Part model, mm, in its own coordinate system. Face numbers are marked on the shaded views. A direction names the side the tool comes from. Round coordinates to 2 decimals unless told otherwise and drop trailing zeros. Write each loop counter-clockwise with the first axis right and the second up, starting at its lowest first coordinate (ties: lowest second). Pieces come first, ordered by that corner, then holes. Notation, with made-up numbers: (-6.75, 47) -> (46.25, 47) arc R18 cw to (46.25, 63) -> close; hole circle Ø9 at (11.5, 66.25). An arc over 180 degrees is marked (long way). Use CSV: the item, a comma, the result in double quotes. Start each with the question number.
(1) Which spindle directions (+Z, -Z, +X, -X, +Y, -Y) get a long thin tool onto all of the face, cutting with end or side? Do the marked faces 1 and 2. Say none if no direction does.
(2) Drop flat-ended pins along their axis: pin 1 (7 mm diameter, centred on x = -14.89, y = -8.6, fed in from -Z); pin 2 (4 mm diameter, centred on x = -14, z = 6.5, fed in from +Y); pin 3 (18 mm diameter, centred on x = -7.5, y = 5.5, fed in from +Z); pin 4 (3 mm diameter, centred on x = 11.5, z = 1.5, fed in from +Y). Give the stop position or say it passes through.
(3) Saw through at D-D (x = 24). Give the cut face in (y, z), plus the area to 3 significant figures.
(4) Saw through at C-C (z = 10). Give the cut face in (x, y), plus the area to 3 significant figures.
(5) Saw through at A-A (y = 0). Give the cut face in (x, z), plus the area to 3 significant figures.
(6) Saw through at B-B (x = 0). Give the cut face in (y, z).
(7) Probe line 1 (Y direction, x = 0, z = 0.55); line 2 (Y direction, x = 6, z = 5.75); line 3 (Z direction, x = 23.5, y = -18.5). List the from-to ranges inside material, lowest first. Write a range as [from, to].
(8) Two-plate mould, pull along X, no slides. Class the marked faces 3, 4, 5 and 6: released by +X, released by -X, zero draft, split by the parting line, or undercut.
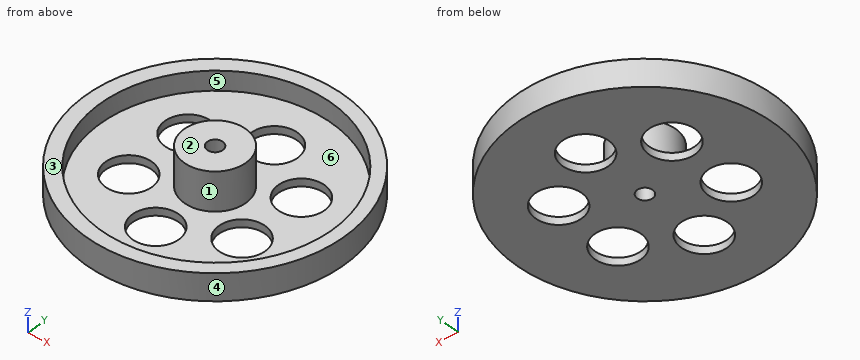
```python
from build123d import *

# Parameters (mm, degrees)
SKETCH1_R           = 33.5
BOSS_EXTRUDE1_DEPTH = 7
SKETCH2_R           = 30
CUT_EXTRUDE1_DEPTH  = 5
SKETCH3_R           = 8
BOSS_EXTRUDE2_DEPTH = 10
SKETCH4_R           = 2
CUT_EXTRUDE2_DEPTH  = 30
SKETCH5_R           = 6
CUT_EXTRUDE3_DEPTH  = 3
CIRPATTERN1_COUNT   = 6


with BuildPart() as part:
    # Sketch1 → Boss-Extrude1 (new body)
    with BuildSketch(Plane.XY):
        Circle(SKETCH1_R)
    extrude(amount=BOSS_EXTRUDE1_DEPTH)

    # Sketch2 → Cut-Extrude1 (cut)
    with BuildSketch(Plane.XY.offset(7)):
        with Locations((0.329125808, 0)):
            Circle(SKETCH2_R)
    extrude(amount=-CUT_EXTRUDE1_DEPTH, mode=Mode.SUBTRACT)

    # Sketch3 → Boss-Extrude2 (add)
    with BuildSketch(Plane.XY.offset(2)):
        Circle(SKETCH3_R)
    extrude(amount=BOSS_EXTRUDE2_DEPTH)

    # Sketch4 → Cut-Extrude2 (cut)
    with BuildSketch(Plane.XY.offset(12)):
        Circle(SKETCH4_R)
    extrude(amount=-CUT_EXTRUDE2_DEPTH, mode=Mode.SUBTRACT)

    # Sketch5 → Cut-Extrude3 (cut, through all)
    with BuildSketch(Plane.XY.offset(2)):
        with Locations((0, 17.196823471)):
            Circle(SKETCH5_R)
    cut_extrude3 = extrude(amount=-CUT_EXTRUDE3_DEPTH, mode=Mode.SUBTRACT)

    # CirPattern1: Cut-Extrude3 ×6 about axis
    cirpattern1_axis = Axis((0, 0, 0), (0, 0, 1))
    for i in range(1, CIRPATTERN1_COUNT):
        add(cut_extrude3.rotate(cirpattern1_axis, i * 360 / CIRPATTERN1_COUNT), mode=Mode.SUBTRACT)


solid = part.part
```
Answers:
1,face 1,"+Z"
1,face 2,"+Z, +X, -X, +Y, -Y"
2,pin 1,"passes through"
2,pin 2,"stops at y = 31.28"
2,pin 3,"stops at z = 12"
2,pin 4,"stops at y = 31.97"
3,outline,"(-23.37, 0) -> (23.37, 0) -> (23.37, 7) -> (18.43, 7) -> (18.43, 2) -> (-18.43, 2) -> (-18.43, 7) -> (-23.37, 7) -> close"
3,area,"143 mm²"
4,outline,"circle Ø16 at (0, 0); hole circle Ø4 at (0, 0)"
4,area,"188 mm²"
5,outline,"(-33.5, 0) -> (-2, 0) -> (-2, 12) -> (-8, 12) -> (-8, 2) -> (-29.67, 2) -> (-29.67, 7) -> (-33.5, 7) -> close; (2, 0) -> (33.5, 0) -> (33.5, 7) -> (30.33, 7) -> (30.33, 2) -> (8, 2) -> (8, 12) -> (2, 12) -> close"
5,area,"281 mm²"
6,outline,"(-33.5, 0) -> (-23.2, 0) -> (-23.2, 2) -> (-30, 2) -> (-30, 7) -> (-33.5, 7) -> close; (-11.2, 0) -> (-2, 0) -> (-2, 12) -> (-8, 12) -> (-8, 2) -> (-11.2, 2) -> close; (2, 0) -> (11.2, 0) -> (11.2, 2) -> (8, 2) -> (8, 12) -> (2, 12) -> close; (23.2, 0) -> (33.5, 0) -> (33.5, 7) -> (30, 7) -> (30, 2) -> (23.2, 2) -> close"
7,line 1,"y = [-33.5, -23.2], [-11.2, -2], [2, 11.2], [23.2, 33.5]"
7,line 2,"y = [-32.96, -29.46], [-5.29, 5.29], [29.46, 32.96]"
7,line 3,"z = [0, 2]"
8,face 3,"zero draft"
8,face 4,"split by the parting line"
8,face 5,"undercut"
8,face 6,"undercut"
